```python
from build123d import *

# Parameters (mm, degrees)
CROQUIS1_W              = 20
CROQUIS1_H              = 60
SALIENTE_EXTRUIR1_DEPTH = 16
CORTAR_EXTRUIR1_DEPTH   = 36.440090293
CROQUIS3_R              = 1.5
CORTAR_EXTRUIR2_DEPTH   = 3
CROQUIS4_R              = 1.5
CORTAR_EXTRUIR3_DEPTH   = 8
REDONDEO1_R             = 5


with BuildPart() as part:
    # Croquis1 → Saliente-Extruir1 (new body)
    with BuildSketch(Plane(origin=(0, 0, 0), x_dir=(1, 0, 0), z_dir=(0, 1, 0))):
        Rectangle(CROQUIS1_W, CROQUIS1_H)
    extrude(amount=SALIENTE_EXTRUIR1_DEPTH)

    # Croquis2 → Cortar-Extruir1 (cut, through all)
    with BuildSketch(Plane(origin=(0, 16, 0), x_dir=(1, 0, 0), z_dir=(0, 1, 0))):
        with BuildLine():
            Line((-3.464101615, 27), (3.464101615, 27))
            ThreePointArc((3.464101615, 27), (6.5, 21.5), (3.464101615, 16))
            Line((3.464101615, 16), (-3.464101615, 16))
            ThreePointArc((-3.464101615, 16), (-6.5, 21.5), (-3.464101615, 27))
        make_face()
    extrude(amount=-CORTAR_EXTRUIR1_DEPTH, mode=Mode.SUBTRACT)

    # Croquis3 → Cortar-Extruir2 (cut)
    with BuildSketch(Plane(origin=(0, 0, -30), x_dir=(-1, 0, 0), z_dir=(0, 0, -1))):
        with Locations((0, 12)):
            Circle(CROQUIS3_R)
        with Locations((0, 4)):
            Circle(CROQUIS3_R)
    extrude(amount=-CORTAR_EXTRUIR2_DEPTH, mode=Mode.SUBTRACT)

    # Croquis4 → Cortar-Extruir3 (cut)
    with BuildSketch(Plane(origin=(0, 16, 0), x_dir=(1, 0, 0), z_dir=(0, 1, 0))):
        with Locations(Location((0, 13, 0), (0, 0, 270))):
            Circle(CROQUIS4_R)
        with Locations(Location((0, 8, 0), (0, 0, 270))):
            Circle(CROQUIS4_R)
        with Locations(Location((0, 3, 0), (0, 0, 270))):
            Circle(CROQUIS4_R)
        with Locations(Location((0, -2, 0), (0, 0, 270))):
            Circle(CROQUIS4_R)
        with Locations(Location((0, -7, 0), (0, 0, 270))):
            Circle(CROQUIS4_R)
        with Locations(Location((0, -12, 0), (0, 0, 270))):
            Circle(CROQUIS4_R)
        with Locations(Location((0, -17, 0), (0, 0, 270))):
            Circle(CROQUIS4_R)
        with Locations(Location((0, -22, 0), (0, 0, 270))):
            Circle(CROQUIS4_R)
        with Locations(Location((0, -27, 0), (0, 0, 270))):
            Circle(CROQUIS4_R)
    extrude(amount=-CORTAR_EXTRUIR3_DEPTH, mode=Mode.SUBTRACT)

    # Redondeo1
    redondeo1_edges = [part.edges().sort_by_distance(p)[0] for p in [
        (-10, 8, -30),
        (10, 8, -30),
    ]]
    fillet(redondeo1_edges, radius=REDONDEO1_R)


solid = part.part
```
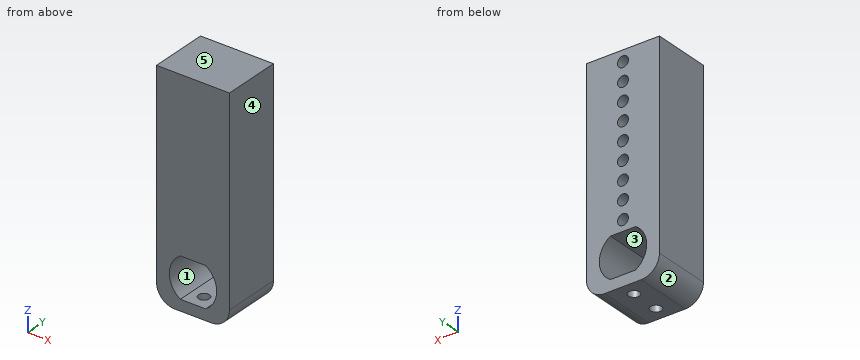
The listing builds one solid part. Answer for the finished solid, in the listing's coordinates (mm). Face numbers are marked on the shaded views. A direction names the side the tool comes from. Give positions to 0.01 mm unless a question says otherwise; leave off trailing zeros. Loops run counter-clockwise (first coordinate to the right, second up) from the corner with the lowest first, then second, coordinate; pieces in that order, holes last. Notation, with made-up numbers: M 3,43 L 15,43 A16 ccw 15,53 Z; hole C 46,39.25 d10. An arc over 180 degrees is marked long. One line per item, written item: value.
1. Section C-C on x = -4 is taken. Determine the outline of the cut face in (y, z), plus the area to 3 significant figures.
Found:
outline: M 0,-30 L 16,-30 L 16,-26.62 L 0,-26.62 Z; M 0,-16.38 L 16,-16.38 L 16,30 L 0,30 Z
area: 796 mm^2
2. For the marked faces 1 and 2, determine the directions among +Z, -Z, +X, -X, +Y, -Y from which every point of the face is accessible in a straight line to the end or side of a thin tool.
Found:
face 1: +Y, -Y
face 2: -Z, -X, +Y, -Y
3. Find the intervals of material crossed by probe 1 along X at (y, z) = (13, 2); probe 2 along Z at (x, y) = (2.5, 1); probe 3 along X at (y, z) = (8.5, -4), in increasing order.
Found:
probe 1: -10 to -1.5, 1.5 to 10
probe 2: -30 to -27, -16 to 30
probe 3: -10 to -1.12, 1.12 to 10
4. Section A-A on y = 14.5 is taken. State how many separate pieces and enclosed holes the cut face has, plus the area to 3 significant figures.
Found:
separate pieces: 1
enclosed holes: 10
area: 1,000 mm^2
5. Section B-B on z = -13 is taken. Determine the outline of the cut face in (x, y).
Found:
outline: M -10,0 L 10,0 L 10,16 L 1.5,16 L 1.5,8 L -1.5,8 L -1.5,16 L -10,16 Z
6. Each of these flat-tipped pins is pushed along its axis until it touches: P1, Ø2.5, axis at x = 0, y = 4, coming from the -Z side; P2, Ø2.5, axis at x = 0, z = 7, coming from the +Y side. Where does it stop, or does it pass through?
Found:
P1: z = -16
P2: y = 8
7. For a pull along X with two mould halves and no side action, classify the marked faces 3, 4 and 5 as pulls with the +X half, pulls with the -X half, needs draft (parallel to the pull), parting line crosses it, or undercut.
Found:
face 3: undercut
face 4: pulls with the +X half
face 5: needs draft
